Source: CAD feature listing. Evaluate the final solid. Frame: model axes, mm. Face numbers are marked on the shaded views. A direction names the side the tool comes from. Coordinates: 2 decimals unless noted, no trailing zeros. Write each loop counter-clockwise with the first axis right and the second up, starting at its lowest first coordinate (ties: lowest second). Pieces come first, ordered by that corner, then holes. Notation, with made-up numbers: M 83,3.25 L 98,3.25 A32 cw 98,42.25 Z; hole C 17,-12.5 d3. An arc over 180 degrees is marked long. Write item = value, one per line. Start each with the question number.
1. Section query B-B (x = -0.1). Output: boundary loops of the cut face in (y, z) (3 decimals).
2. Line query: line 1 along Z through (x, y) = (0.1, 1.1); line 2 along Z through (x, y) = (0.9, 0.4); line 3 along Z through (x, y) = (0.2, 2). Output: solid intervals per line, ascending.
3. Section query A-A (y = 2.35). Output: boundary loops of the cut face in (x, z) (3 decimals).
4. Access query for the marked faces 4, 5, 6, 7 and 8. Directions: +Z, -Z, +X, -X, +Y, -Y. A direction counts if a zero-diameter tool reaches every point of the face in a straight line with its end or side. Return the directions, or none.
5. Pull-direction query (Z, two-part tool) for the marked faces 1, 2 and 3; classes: pulls with the +Z half, pulls with the -Z half, needs draft (parallel to the pull), parting line crosses it, or undercut.
6. Pin query (flat end, axial travel): pin 1 Ø0.7 at (y, z) = (0.5, 3) entering from +X; pin 2 Ø1 at (y, z) = (2, 2) entering from -X. Return the tip coordinate at first contact, or that it passes through.
7. Section query C-C (y = 0.65). Output: boundary loops of the cut face in (x, z) (3 decimals).
8. Section query D-D (z = 0). Output: boundary loops of the cut face in (x, y) (3 decimals).
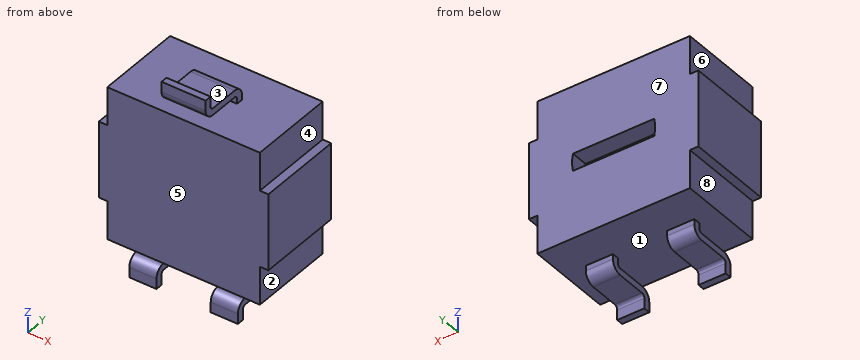
```python
from build123d import *

# Parameters (mm, degrees)
SKETCH1_W                                      = 4.5
SKETCH1_H                                      = 4.5
BASE_EXTRUDE_DEPTH                             = 2.55
SKETCH2_W                                      = 0.25
SKETCH2_H                                      = 2.25
EARS_EXTRUDE1_DEPTH                            = 2.55
DOUBLE_START                                   = -1.6
DOUBLE_FEET_EXTRUDE_THIN1_DEPTH                = 3.2
SINGLE_START                                   = -0.65
SINGLE_FOOT_EXTRUDE_THIN2_DEPTH                = 1.3
SKETCH5_W                                      = 1.6
SKETCH5_H                                      = 0.85
REMOVE_MIDDLE_OF_THE_DOUBLE_PINS_EXTRUDE_DEPTH = 5.728900506
SCREW_DRIVER_SLOT_EXTRUDE2_DEPTH               = 0.51


# Read off the part's stored shape, not the designer's step: double feet-Extrude-Thin1, single foot-Extrude-Thin2
with BuildPart() as part:
    # Sketch1 → Base-Extrude (new body)
    with BuildSketch(Plane(origin=(0, 0, 0), x_dir=(1, 0, 0), z_dir=(0, 1, 0))):
        Rectangle(SKETCH1_W, SKETCH1_H)
    extrude(amount=BASE_EXTRUDE_DEPTH)

    # Sketch2 → ears-Extrude1 (add, through all)
    with BuildSketch(Plane(origin=(0, 2.55, 0), x_dir=(-1, 0, 0), z_dir=(0, 1, 0))):
        with Locations((-2.375, 0)):
            Rectangle(SKETCH2_W, SKETCH2_H)
        with Locations((2.375, 0)):
            Rectangle(SKETCH2_W, SKETCH2_H)
    extrude(amount=-EARS_EXTRUDE1_DEPTH)

    # double feet-Extrude-Thin1 outline → double feet-Extrude-Thin1 (add)
    with BuildSketch(Plane(origin=(0, 0, 0), x_dir=(0, 0, -1), z_dir=(1, 0, 0)).offset(DOUBLE_START)):
        with BuildLine():
            ThreePointArc((2.5, 0.3), (2.587867966, 0.087867966), (2.8, 0))
            Line((2.8, 0), (3.1, 0))
            Line((3.1, 0), (3.1, 0.2))
            Line((3.1, 0.2), (2.8, 0.2))
            ThreePointArc((2.8, 0.2), (2.729289322, 0.229289322), (2.7, 0.3))
            Line((2.7, 0.3), (2.7, 1.175))
            ThreePointArc((2.7, 1.175), (2.612132034, 1.387132034), (2.4, 1.475))
            Line((2.4, 1.475), (2.25, 1.475))
            Line((2.25, 1.475), (2.25, 1.275))
            Line((2.25, 1.275), (2.4, 1.275))
            ThreePointArc((2.4, 1.275), (2.470710678, 1.245710678), (2.5, 1.175))
            Line((2.5, 1.175), (2.5, 0.3))
        make_face()
    extrude(amount=DOUBLE_FEET_EXTRUDE_THIN1_DEPTH)

    # single foot-Extrude-Thin2 outline → single foot-Extrude-Thin2 (add)
    with BuildSketch(Plane(origin=(0, 0, 0), x_dir=(0, 0, -1), z_dir=(1, 0, 0)).offset(SINGLE_START)):
        with BuildLine():
            Line((-3.1, 0), (-2.8, 0))
            ThreePointArc((-2.8, 0), (-2.587867966, 0.087867966), (-2.5, 0.3))
            Line((-2.5, 0.3), (-2.5, 1.175))
            ThreePointArc((-2.5, 1.175), (-2.470710678, 1.245710678), (-2.4, 1.275))
            Line((-2.4, 1.275), (-2.25, 1.275))
            Line((-2.25, 1.275), (-2.25, 1.475))
            Line((-2.25, 1.475), (-2.4, 1.475))
            ThreePointArc((-2.4, 1.475), (-2.612132034, 1.387132034), (-2.7, 1.175))
            Line((-2.7, 1.175), (-2.7, 0.3))
            ThreePointArc((-2.7, 0.3), (-2.729289322, 0.229289322), (-2.8, 0.2))
            Line((-2.8, 0.2), (-3.1, 0.2))
            Line((-3.1, 0.2), (-3.1, 0))
        make_face()
    extrude(amount=SINGLE_FOOT_EXTRUDE_THIN2_DEPTH)

    # Sketch5 → remove middle of the double pins-Extrude1 (cut, through all)
    with BuildSketch(Plane(origin=(0, 2.55, 0), x_dir=(-1, 0, 0), z_dir=(0, 1, 0))):
        with Locations((0, -2.675)):
            Rectangle(SKETCH5_W, SKETCH5_H)
    extrude(amount=-REMOVE_MIDDLE_OF_THE_DOUBLE_PINS_EXTRUDE_DEPTH, mode=Mode.SUBTRACT)

    # Sketch7 → screw driver slot-Extrude2 (cut)
    with BuildSketch(Plane(origin=(0, 2.55, 0), x_dir=(-1, 0, 0), z_dir=(0, 1, 0))):
        with BuildLine():
            Line((-1.198165264, 0.255), (1.198165264, 0.255))
            ThreePointArc((1.198165264, 0.255), (1.225, 0), (1.198165264, -0.255))
            Line((1.198165264, -0.255), (-1.198165264, -0.255))
            ThreePointArc((-1.198165264, -0.255), (-1.225, 0), (-1.198165264, 0.255))
        make_face()
    extrude(amount=-SCREW_DRIVER_SLOT_EXTRUDE2_DEPTH, mode=Mode.SUBTRACT)


solid = part.part
```
Results are:
q1.outline = M 0,-2.25 L 2.55,-2.25 L 2.55,-0.255 L 2.04,-0.255 L 2.04,0.255 L 2.55,0.255 L 2.55,2.25 L 1.475,2.25 L 1.475,2.4 A0.3 ccw 1.175,2.7 L 0.3,2.7 A0.1 cw 0.2,2.8 L 0.2,3.1 L 0,3.1 L 0,2.8 A0.3 ccw 0.3,2.5 L 1.175,2.5 A0.1 cw 1.275,2.4 L 1.275,2.25 L 0,2.25 Z
q2.line_1 = -2.25 to 2.25, 2.5 to 2.7
q2.line_2 = -2.7 to -2.5, -2.25 to 2.25
q2.line_3 = -2.25 to 2.25
q3.outline = M -2.5,-1.125 L -2.25,-1.125 L -2.25,-2.25 L 2.25,-2.25 L 2.25,-1.125 L 2.5,-1.125 L 2.5,1.125 L 2.25,1.125 L 2.25,2.25 L -2.25,2.25 L -2.25,1.125 L -2.5,1.125 Z; hole M -1.198,-0.255 L 1.198,-0.255 A1.225 ccw 1.198,0.255 L -1.198,0.255 A1.225 ccw Z
q4.face_4 = +Z, +X, +Y, -Y
q4.face_5 = +Z, -Z, +X, -X, -Y
q4.face_6 = +Z, -X, +Y, -Y
q4.face_7 = +Z, -Z, +X, -X, +Y
q4.face_8 = -Z, -X, +Y, -Y
q5.face_1 = undercut
q5.face_2 = needs draft
q5.face_3 = pulls with the +Z half
q6.pin_1 = 0.65
q6.pin_2 = -2.25
q7.outline = M -2.5,-1.125 L -2.25,-1.125 L -2.25,-2.25 L 2.25,-2.25 L 2.25,-1.125 L 2.5,-1.125 L 2.5,1.125 L 2.25,1.125 L 2.25,2.25 L -2.25,2.25 L -2.25,1.125 L -2.5,1.125 Z; M -1.6,-2.7 L -0.8,-2.7 L -0.8,-2.5 L -1.6,-2.5 Z; M -0.65,2.5 L 0.65,2.5 L 0.65,2.7 L -0.65,2.7 Z; M 0.8,-2.7 L 1.6,-2.7 L 1.6,-2.5 L 0.8,-2.5 Z
q8.outline = M -2.5,0 L 2.5,0 L 2.5,2.55 L 1.225,2.55 L 1.225,2.04 L -1.225,2.04 L -1.225,2.55 L -2.5,2.55 Z
